Autodesk Inventor part; units mm, degrees
ref_plane "YZ Plane" through (0, 0, 0) normal (1, 0, 0) x (0, 1, 0)
ref_plane "XZ Plane" through (0, 0, 0) normal (0, 1, 0) x (-1, 0, 0)
ref_plane "XY Plane" through (0, 0, 0) normal (0, 0, 1) x (1, 0, 0)
sketch "스케치4" plane through (0, 0, 0) normal (0, 0, 1) x (1, 0, 0)
  circle A0 centre (264.0912, 143.5876) radius 1.9
  circle A1 centre (235.6112, 63.5885) radius 1.9
  circle A2 centre (292.5662, 63.5867) radius 1.9
  circle A3 centre (264.0899, 46.4242) radius 3.75
  circle A4 centre (264.0899, 102.1242) radius 33.15
  circle A5 centre (292.5662, 63.5867) radius 1.5
  circle A6 centre (235.6112, 63.5885) radius 1.5
  circle A7 centre (264.0912, 143.5876) radius 1.5
  line L0 (264.0899, 102.1242) -> (264.0899, 46.4242)
  line L1 (356.232, 0) -> (158.7026, 0)
  circle A8 centre (264.0912, -143.5876) radius 1.9
  circle A9 centre (235.6112, -63.5885) radius 1.9
  circle A10 centre (292.5662, -63.5867) radius 1.9
  circle A11 centre (264.0899, -46.4242) radius 3.75
  circle A12 centre (264.0899, -102.1242) radius 33.15
  circle A13 centre (235.6112, -63.5885) radius 1.5
  circle A14 centre (264.0912, -143.5876) radius 1.5
  circle A15 centre (292.5662, -63.5867) radius 1.5
  line L2 (264.0899, -102.1242) -> (264.0899, -46.4242) construction
  line L3 (320.9052, -28.3469) -> (207.2359, -28.3469)
  line L4 (207.2359, -28.3469) -> (207.2359, -169.6626)
  line L5 (207.2359, -169.6626) -> (320.9052, -169.6626)
  line L6 (320.9052, -169.6626) -> (320.9052, -28.3469)
  point P0 (0, 0)
  dimension "d38" = 3
  dimension "d39" = 3
  dimension "d40" = 3
  dimension "d41" = 41.4634
  dimension "d42" = 47.917
  dimension "d45" = 7.5
  dimension "d48" = 143.537
  dimension "d50" = 47.917
  dimension "d51" = 36.465
  dimension "d52" = 36.462
  dimension "d53" = 179.998
  dimension "d54" = 55.7
extrude "돌출3" add sketch "스케치4" along normal blind 10 contours L6 L5 L4 L3
properties part number "Lidar"
Here's how the part is built. I have some questions about the finished solid (model axes, mm). Coordinates: 2 decimals unless noted, no trailing zeros. Order: outer loops, then holes, each group sorted by start corner. A loop starts at its lowest first (then second) coordinate and runs counter-clockwise, first axis right, second up.
Item 1: If we section it at D-D, the plane x = 264.5: List the corners of the cut face in (y, z) for me, then the cut area to 3 significant figures.
Response values:
outline: (-169.66, 0) - (-145.44, 0) - (-145.44, 10) - (-169.66, 10) - close; (-141.73, 0) - (-135.27, 0) - (-135.27, 10) - (-141.73, 10) - close; (-68.98, 0) - (-50.15, 0) - (-50.15, 10) - (-68.98, 10) - close; (-42.7, 0) - (-28.35, 0) - (-28.35, 10) - (-42.7, 10) - close
area: 639 mm2
Item 2: If we section it at A-A, the plane y = -85: List the corners of the cut face in (x, z) for me.
Response values:
outline: (207.24, 0) - (235.71, 0) - (235.71, 10) - (207.24, 10) - close; (292.47, 0) - (320.91, 0) - (320.91, 10) - (292.47, 10) - close
Item 3: I need wall thicknesses on probe 1 along X at (y, z) = (-101, 1.5); probe 2 along X at (y, z) = (-62, 5.75); probe 3 along Y at (x, z) = (260, 9.25). Which ranges of each line are inside material? Lowest first, please.
Response values:
probe 1: x = 207.24 to 230.96, 297.22 to 320.91
probe 2: x = 207.24 to 234.57, 236.65 to 291.52, 293.61 to 320.91
probe 3: y = -169.66 to -135.02, -69.23 to -28.35
Item 4: Thinking about a two-plate mould opening in Y: for faces 1 (the face through (265, -28.347, 5)), 2 (the face through (207.236, -98, 5)), 3 (the face through (239.66, -124.53, 4.93)), which applies, pulls with the +Y half, pulls with the -Y half, needs draft (parallel to the pull), parting line crosses it, or undercut?
Response values:
face 1: pulls with the +Y half
face 2: needs draft
face 3: undercut
Item 5: If we section it at B-B, the plane z = 3.75: List the corners of the cut face in (x, y) for me.
Response values:
outline: (207.24, -169.66) - (320.91, -169.66) - (320.91, -28.35) - (207.24, -28.35) - close; hole circle Ø66.3 at (264.09, -102.12); hole circle Ø3.8 at (235.61, -63.59); hole circle Ø7.5 at (264.09, -46.42); hole circle Ø3.8 at (264.09, -143.59); hole circle Ø3.8 at (292.57, -63.59)
Item 6: If we section it at C-C, the plane x = 249.5: List the corners of the cut face in (y, z) for me, then the cut area to 3 significant figures.
Response values:
outline: (-169.66, 0) - (-131.89, 0) - (-131.89, 10) - (-169.66, 10) - close; (-72.36, 0) - (-28.35, 0) - (-28.35, 10) - (-72.36, 10) - close
area: 818 mm2
